Design review of the part built by this model. Coordinates are the model's own, in mm. A direction names the side the tool comes from. Give positions to 0.01 mm unless a question says otherwise; leave off trailing zeros. Use one line per item in the form item = value. Start each with the question number.
from build123d import *

# Parameters (mm, degrees)
SHELL_1_T       = -2
SKETCH_4_R      = 7.385297863
EXTRUDE_1_DEPTH = 25
FILLET_1_R      = 4
SKETCH_5_R      = 2.277696926
EXTRUDE_2_DEPTH = 10


with BuildPart() as part:
    # 草图2 → 旋转1 (revolve)
    with BuildSketch(Plane.XY, mode=Mode.PRIVATE) as revolve_1_sk:
        with BuildLine():
            Line((0, 0), (29.253375884, 0))
            ThreePointArc((29.253375884, 0), (22.447823433, 17.880245703), (7.385297863, 29.675967555))
            Line((7.385297863, 29.675967555), (0, 29.675967555))
            Line((0, 29.675967555), (0, 0))
        make_face()
    revolve(revolve_1_sk.sketch.rotate(Axis((0, 0, 0), (0, 1, 0)), 90), axis=Axis((0, 0, 0), (0, 1, 0)))

    # 抽壳1
    shell_1_openings = [part.faces().sort_by_distance(p)[0] for p in [
        (0, 0, 0),
    ]]
    offset(amount=SHELL_1_T, openings=shell_1_openings, kind=Kind.INTERSECTION)

    # 草图4 → 凸台-拉伸1 (add)
    with BuildSketch(Plane(origin=(0, 29.675967555, 0), x_dir=(1, 0, 0), z_dir=(0, 1, 0))):
        with Locations(Location((0, 0, 0), (0, 0, 270))):
            Circle(SKETCH_4_R)
    extrude(amount=EXTRUDE_1_DEPTH)

    # 圆角1
    fillet_1_edges = [part.edges().sort_by_distance(p)[0] for p in [
        (0, 54.675967555, -7.385297863),
    ]]
    fillet(fillet_1_edges, radius=FILLET_1_R)

    # 草图5 → 凸台-拉伸2 (add)
    with BuildSketch(Plane(origin=(0, 0, 0), x_dir=(0, 0, -1), z_dir=(1, 0, 0))):
        with Locations(Location((0, 42.315325321, 0), (0, 0, 180))):
            Circle(SKETCH_5_R)
    extrude(amount=EXTRUDE_2_DEPTH)


solid = part.part
1. Draft analysis for pull direction X (two halves, no side actions). For faces 1 (the flat face through (0, 27.676, 0)), 2 (the flat face through (26, 0, -9)), 3 (the cylindrical face through (-7.21, 40.03, -1.6)), state which applies: pulls with the +X half, pulls with the -X half, needs draft (parallel to the pull), parting line crosses it, or undercut.
2. To check wall thickness, follow L1, parallel to Z at x = -7.5, y = 16; L2, parallel to X at y = 9.5, z = -2; L3, parallel to Z at x = -15.5, y = 16. State the ranges of each line that lie inside material, in increasing order.
3. Clearance check with flat-ended pins moving along their axes: pin 1 Ø4 at (y, z) = (15.5, -8) entering from -X; pin 2 Ø1.5 at (x, z) = (-14.5, -16.5) entering from +Y; pin 3 Ø12 at (x, y) = (-17, 32.5) entering from +Z; pin 4 Ø7 at (x, z) = (-0.5, 2) entering from -Y. State where each tip first meets the part, or that it passes through.
4. For faces 4 (the flat face through (0, 54.676, 0)), 5 (the cylindrical face through (8.487, 44.336, 1.051)), 6 (the flat face through (10, 42, 0)), list the 3-axis set-ups (+Z, -Z, +X, -X, +Y, -Y) from which the entire face can be reached by the end or side of a thin tool; tool diameter is ignored.
Answer block:
q1.face_1 = undercut
q1.face_2 = needs draft
q1.face_3 = parting line crosses it
q2.L1 = -22.53 to -19.97, 19.97 to 22.53
q2.L2 = -26.96 to -24.8, 24.8 to 26.96
q2.L3 = -17.99 to -14.66, 14.66 to 17.99
q3.pin_1 = -24.07
q3.pin_2 = 19.46
q3.pin_3 = through
q3.pin_4 = 27.68
q4.face_4 = +Z, -Z, +X, -X, +Y
q4.face_5 = +X
q4.face_6 = +Z, -Z, +X, +Y
